Job drawing, mm, ordinate dimensions from the low corner. One solid piece. A direction names the side the tool comes from. Give positions to 0.01 mm unless a question says otherwise; leave off trailing zeros. Write each loop counter-clockwise with the first axis right and the second up, starting at its lowest first coordinate (ties: lowest second). Pieces come first, ordered by that corner, then holes. Notation, with made-up numbers: (84.5, -36.5) - (114.5, -36.5) arc R17 cw to (114.5, -24.5) - close; hole circle Ø5 at (-9, 66). An arc over 180 degrees is marked (long way). Answer as a JSON object with one key per item and string values.
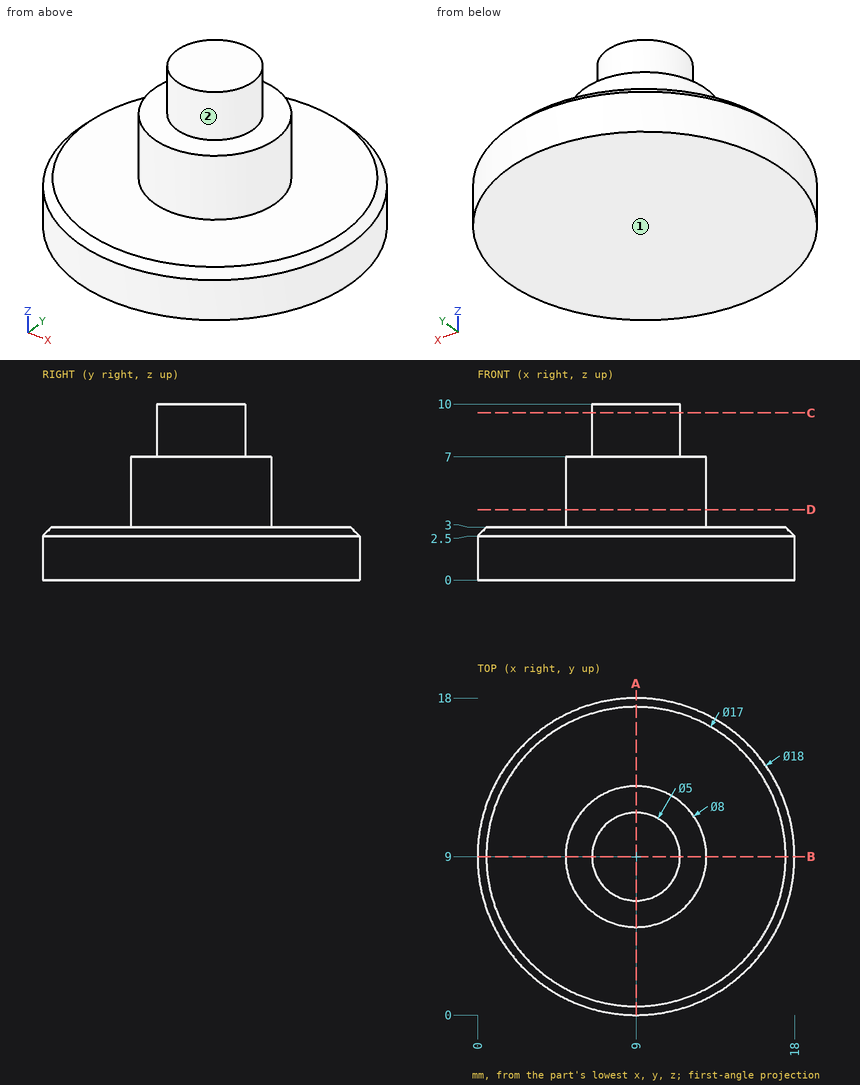
Item 1: Cut at D-D (z = 4). Give the cut face in (x, y), and give its area (3 significant figures).
Entries:
{"outline": "circle Ø8 at (9, 9)", "area": "50.3 mm2"}
Item 2: Which spindle directions (+Z, -Z, +X, -X, +Y, -Y) get a long thin tool onto all of the face, cutting with end or side? Do the marked faces 1 and 2. Say none if no direction does.
Entries:
{"face 1": "-Z, +X, -X, +Y, -Y", "face 2": "+Z"}
Item 3: Probe line 1 (Z direction, x = 11.5, y = 16.5); line 2 (Y direction, x = 12.25, z = 1); line 3 (Y direction, x = 13.75, z = 1). List the from-to ranges inside material, lowest first. Write a range as from..to.
Entries:
{"line 1": "0..3", "line 2": "0.61..17.39", "line 3": "1.36..16.64"}
Item 4: Flat gauge pins, fed straight in: P1, Ø6, axis at x = 12, z = 4, coming from the -Y side; P2, Ø1, axis at y = 15, z = 5.5, coming from the +X side; P3, Ø6, axis at y = 7.5, z = 8, coming from the -X side. Where does each tip first touch, or does it go through?
Entries:
{"P1": "y = 0.01", "P2": "through", "P3": "x = 5"}
Item 5: Cut at A-A (x = 9). Give the cut face in (y, z).
Entries:
{"outline": "(0, 0) - (18, 0) - (18, 2.5) - (17.5, 3) - (13, 3) - (13, 7) - (11.5, 7) - (11.5, 10) - (6.5, 10) - (6.5, 7) - (5, 7) - (5, 3) - (0.5, 3) - (0, 2.5) - close"}
Item 6: Cut at C-C (z = 9.5). Give the cut face in (x, y).
Entries:
{"outline": "circle Ø5 at (9, 9)"}
